Check sheet for the modelled part. Datum: model origin and axes. Units: mm. Face numbers are marked on the shaded views. Coordinates: 2 decimals unless noted, no trailing zeros. Loops run counter-clockwise (first coordinate to the right, second up) from the corner with the lowest first, then second, coordinate; pieces in that order, holes last. Notation, with made-up numbers: (-21, 70.5) -> (23, 70.5) arc R36 cw to (23, 105.5) -> close; hole circle Ø1 at (-34, -10.5). An arc over 180 degrees is marked (long way). Use one line per item in the form item = value.
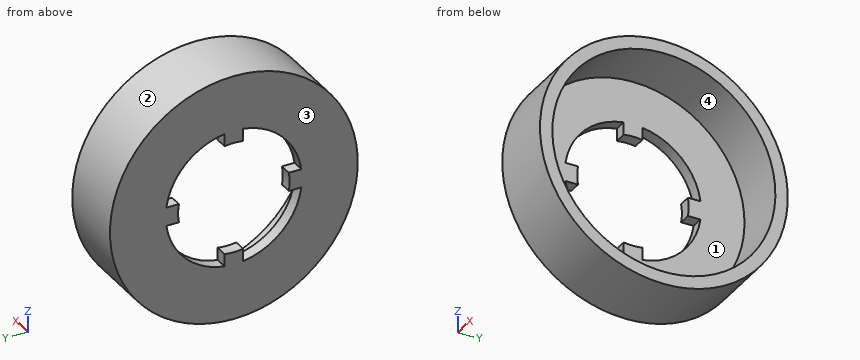
from build123d import *

# Parameters (mm, degrees)
ENL_V_MAT_EXTRU_1_DEPTH = 61.695963622


with BuildPart() as part:
    # Esquisse1 → Base-Révolution (revolve)
    with BuildSketch(Plane.XY, mode=Mode.PRIVATE) as base_r_volution_sk:
        Polygon((0, 40), (0, 18), (4, 18), (4, 36), (22, 36), (22, 40), align=None)
    revolve(base_r_volution_sk.sketch.rotate(Axis((0, 0, 0), (1, 0, 0)), 90), axis=Axis((0, 0, 0), (1, 0, 0)))

    # Esquisse2 → Enlèv. mat.-Extru.1 (cut, through all)
    with BuildSketch(Plane.ZY):
        with BuildLine():
            Line((-3, 16), (-3, 21.794494718))
            ThreePointArc((-3, 21.794494718), (-15.556349186, 15.556349186), (-21.794494718, 3))
            Line((-21.794494718, 3), (-16, 3))
            Line((-16, 3), (-16, -3))
            Line((-16, -3), (-21.794494718, -3))
            ThreePointArc((-21.794494718, -3), (-15.556349186, -15.556349186), (-3, -21.794494718))
            Line((-3, -21.794494718), (-3, -16))
            Line((-3, -16), (3, -16))
            Line((3, -16), (3, -21.794494718))
            ThreePointArc((3, -21.794494718), (15.556349186, -15.556349186), (21.794494718, -3))
            Line((21.794494718, -3), (16, -3))
            Line((16, -3), (16, 3))
            Line((16, 3), (21.794494718, 3))
            ThreePointArc((21.794494718, 3), (15.556349186, 15.556349186), (3, 21.794494718))
            Line((3, 21.794494718), (3, 16))
            Line((3, 16), (-3, 16))
        make_face()
    extrude(amount=-ENL_V_MAT_EXTRU_1_DEPTH, mode=Mode.SUBTRACT)


solid = part.part
(1) Scan lines: line 1 along Y through (x, z) = (15.75, 0); line 2 along X through (y, z) = (-25, 11); line 3 along Y through (x, z) = (15.75, 24). Record each from-to range of solid material in increasing order.
Established:
line_1 = -40 to -36, 36 to 40
line_2 = 0 to 4
line_3 = -32 to -26.83, 26.83 to 32
(2) Go/stop test with flat-tipped pins: P1, Ø1, axis at x = 12, y = -28, coming from the -Z side; P2, Ø4.5, axis at x = 2.5, y = 20.5, coming from the -Z side; P3, Ø3, axis at x = 3, z = 20, coming from the -Y side. Record where each tip stops, or that it passes through.
Established:
P1 = -29.05
P2 = -35.59
P3 = -35.46
(3) Section check C-C, the plane y = -33. Record the boundary of the cut face in (x, z), plus the area to 3 significant figures.
Established:
outline = (0, -22.61) -> (22, -22.61) -> (22, -14.39) -> (4, -14.39) -> (4, 14.39) -> (22, 14.39) -> (22, 22.61) -> (0, 22.61) -> close
area = 477 mm²
(4) Section check D-D, the plane z = 24.5. Record the boundary of the cut face in (x, y), plus the area to 3 significant figures.
Established:
outline = (0, -31.62) -> (22, -31.62) -> (22, -26.38) -> (4, -26.38) -> (4, 26.38) -> (22, 26.38) -> (22, 31.62) -> (0, 31.62) -> close
area = 442 mm²
(5) Mould release check, pull along Y, two halves, no side actions. Record for the marked faces 1, 2, 3 and 4: +Y half, -Y half, draft (parallel to the pull), parting line (faces both ways), or undercut.
Established:
face_1 = undercut
face_2 = parting line
face_3 = draft
face_4 = undercut
(6) Section check A-A, the plane z = 0. Record the boundary of the cut face in (x, y), plus the area to 3 significant figures.
Established:
outline = (0, -40) -> (22, -40) -> (22, -36) -> (4, -36) -> (4, -18) -> (0, -18) -> close; (0, 18) -> (4, 18) -> (4, 36) -> (22, 36) -> (22, 40) -> (0, 40) -> close
area = 320 mm²
